```python
from build123d import *

# Parameters (mm, degrees)
BOSS_EXTRUDE1_DEPTH       = 35.56
CORTAR_EXTRUIR1_DEPTH     = 12.7
CORTAR_EXTRUIR2_DEPTH     = 12.7
CROQUIS4_R                = 6.35
CORTAR_EXTRUIR3_DEPTH     = 35.56
SIMETR_A7_COPY_1_SKETCH_R = 6.35
SIMETR_A7_COPY_1_DEPTH    = 35.56
REDONDEO1_R               = 17.78


with BuildPart() as part:
    # Sketch1 → Boss-Extrude1 (new body)
    with BuildSketch(Plane(origin=(0, 0, 0), x_dir=(1, 0, 0), z_dir=(0, 1, 0))):
        Polygon((47.97173767, 52.13499004), (20.15284418, 0), (47.971737664, -52.13499003), (16.598657301, -68.875462799), (0, -37.768156774), (-16.598657301, -68.875462799), (-32.285197483, -60.505226415), (-47.971737664, -52.13499003), (-20.15284418, 0), (-47.971737664, 52.13499003), (-32.285197483, 60.505226415), (-16.598657301, 68.875462799), (0, 37.768156774), (16.598657296, 68.875462789), (32.28519748, 60.505226416), align=None)
    extrude(amount=BOSS_EXTRUDE1_DEPTH)

    # Croquis2 → Cortar-Extruir1 (cut, symmetric)
    with BuildSketch(Plane(origin=(0, 0, 0), x_dir=(-0.470766951, 0, 0.882257603), z_dir=(-0.882257603, 0, -0.470766951))):
        with BuildLine():
            Line((55.88, 30.48), (68.58, 30.48))
            Line((68.58, 30.48), (68.58, 0))
            Line((68.58, 0), (43.18, 0))
            Line((43.18, 0), (43.18, 17.78))
            ThreePointArc((43.18, 17.78), (46.899743879, 26.760256121), (55.88, 30.48))
        make_face()
    cortar_extruir1 = extrude(amount=CORTAR_EXTRUIR1_DEPTH, both=True, mode=Mode.SUBTRACT)

    # Croquis3 → Cortar-Extruir2 (cut, symmetric)
    with BuildSketch(Plane(origin=(0, 0, 0), x_dir=(-0.470766951, 0, -0.882257603), z_dir=(0.882257603, 0, -0.470766951))):
        with BuildLine():
            Line((-55.88, 30.48), (-68.58, 30.48))
            Line((-68.58, 30.48), (-68.58, 0))
            Line((-68.58, 0), (-43.18, 0))
            Line((-43.18, 0), (-43.18, 17.78))
            ThreePointArc((-43.18, 17.78), (-46.899743879, 26.760256121), (-55.88, 30.48))
        make_face()
    cortar_extruir2 = extrude(amount=CORTAR_EXTRUIR2_DEPTH, both=True, mode=Mode.SUBTRACT)

    # Simetría1: Cortar-Extruir1, Cortar-Extruir2 across plane
    add(cortar_extruir1.mirror(Plane.XY), mode=Mode.SUBTRACT)
    add(cortar_extruir2.mirror(Plane.XY), mode=Mode.SUBTRACT)

    # Croquis4 → Cortar-Extruir3 (cut)
    with BuildSketch(Plane(origin=(-15.686540182, 0, -8.370236384), x_dir=(-0.470766951, 0, 0.882257603), z_dir=(-0.882257603, 0, -0.470766951))):
        with Locations((55.88, 17.78)):
            Circle(CROQUIS4_R)
    cortar_extruir3 = extrude(amount=-CORTAR_EXTRUIR3_DEPTH, mode=Mode.SUBTRACT)

    # Simetría2: Cortar-Extruir3 across plane
    add(cortar_extruir3.mirror(Plane(origin=(0, 0, 0), x_dir=(0, 0, 1), z_dir=(1, 0, 0))), mode=Mode.SUBTRACT)

    # Simetría7: Cortar-Extruir3 across plane
    add(cortar_extruir3.mirror(Plane.XY), mode=Mode.SUBTRACT)

    # Simetría7 copy 1 sketch → Simetría7 copy 1 (cut)
    with BuildSketch(Plane(origin=(15.686540182, 0, 8.370236384), x_dir=(0.470766951, 0, -0.882257603), z_dir=(0.882257603, 0, 0.470766951))):
        with Locations((55.88, 17.78)):
            Circle(SIMETR_A7_COPY_1_SKETCH_R)
    extrude(amount=-SIMETR_A7_COPY_1_DEPTH, mode=Mode.SUBTRACT)

    # Redondeo1
    redondeo1_edges = [part.edges().sort_by_distance(p)[0] for p in [
        (18.839591613, 0, 67.679714744),
        (-45.730803353, 0, 53.330738085),
        (-18.839591613, 0, -67.679714744),
        (45.730803357, 0, -53.330738094),
        (-18.839591613, 0, 67.679714744),
        (45.730803353, 0, 53.330738085),
        (-45.730803353, 0, -53.330738085),
        (18.839591608, 0, -67.679714736),
    ]]
    fillet(redondeo1_edges, radius=REDONDEO1_R)


solid = part.part
```
Read the model definition and answer for the solid it produces. Units are mm, in the model's axes. A direction names the side the tool comes from. Give positions to 0.01 mm unless a question says otherwise; leave off trailing zeros. Loops run counter-clockwise (first coordinate to the right, second up) from the corner with the lowest first, then second, coordinate; pieces in that order, holes last.
Item 1: The part is cut by section C-C (y = 3). Write down the section's boundary in (x, z).
Item 2: The part is cut by section B-B (z = 21). Write down the section's boundary in (x, y), and give its area (3 significant figures).
Item 3: For faces 1 (the cylindrical face through (43.38, 5.35, -48.84)), 2 (the cylindrical face through (42.635, 19.687, -47.453)), 3 (the flat face through (34.257, 17.531, -26.432)), 4 (the flat face through (6.57, 17.53, 50.08)), 5 (the cylindrical face through (-22.189, 26.661, -41.207)), determine the directions among +Z, -Z, +X, -X, +Y, -Y from which every point of the face is accessible in a straight line to the end or side of a thin tool.
Item 4: The mould has two halves that part along X. Classify faces 6 (the cylindrical face through (16.29, 5.07, 62.98)), 7 (the flat face through (29, 30.48, 55)), 8 (the cylindrical face through (-16.29, 5.07, -62.98)): released by +X, released by -X, zero draft, split by the parting line, or undercut.
Item 5: Find the intervals of material crossed by line 1 along X through (y, z) = (8.5, -46.5); line 2 along Z through (x, y) = (-18.5, 28); line 3 along X through (y, z) = (25.5, 44.5), in increasing order.
Item 6: The part is cut by section D-D (z = 58.5). Give the number of separate pieces and of enclosed holes in the cut face, and give its area (3 significant figures).
Item 7: Each of these flat-tipped pins is pushed along its axis until it touches: pin 1 Ø4 at (x, y) = (23.5, 5.5) entering from -Z; pin 2 Ø1 at (y, z) = (22, -5.5) entering from +X; pin 3 Ø18.5 at (x, z) = (-35.5, -49.5) entering from -Y; pin 4 Ø1 at (x, z) = (-29.5, 13.5) entering from -Y. Where does it stop, or does it pass through?
Item 8: The part is cut by section A-A (y = 32.5). Write down the section's boundary in (x, z) (3 decimals).
Taken from the geometry:
1. outline: (-44.25, -45.17) - (-39.77, -47.56) - (-31.53, -32.12) - (-9.12, -44.07) - (-17.36, -59.52) - (-12.88, -61.91) - (0, -37.77) - (12.88, -61.91) - (17.36, -59.52) - (9.12, -44.07) - (31.53, -32.12) - (39.77, -47.56) - (44.25, -45.17) - (20.15, 0) - (44.25, 45.17) - (39.77, 47.56) - (31.53, 32.12) - (9.12, 44.07) - (17.36, 59.52) - (12.88, 61.91) - (0, 37.77) - (-12.88, 61.91) - (-17.36, 59.52) - (-9.12, 44.07) - (-31.53, 32.12) - (-39.77, 47.56) - (-44.25, 45.17) - (-20.15, 0) - close
2. outline: (-31.36, 0) - (31.36, 0) - (31.36, 35.56) - (-31.36, 35.56) - close
2. area: 2,230 mm2
3. face 1: -Z, +X, -Y
3. face 2: none
3. face 3: +X, +Y, -Y
3. face 4: +Z, +Y, -Y
3. face 5: -Y
4. face 6: released by +X
4. face 7: undercut
4. face 8: released by -X
5. line 1: x = -44.96 to -39.21, -10.42 to -4.66, 4.66 to 10.42, 39.21 to 44.96
5. line 2: z = -67.86 to -61.65, -44.92 to 44.92, 61.65 to 67.86
5. line 3: x = -43.9 to -38.14, -13.88 to -3.59, 3.59 to 13.88, 38.14 to 43.9
6. separate pieces: 4
6. enclosed holes: 0
6. area: 451 mm2
7. pin 1: stops at z = -37.47
7. pin 2: stops at x = 23.35
7. pin 3: stops at y = 0.07
7. pin 4: passes through
8. outline: (-47.972, -52.135) - (-16.599, -68.875) - (0, -37.768) - (16.599, -68.875) - (47.972, -52.135) - (20.153, 0) - (47.972, 52.135) - (16.599, 68.875) - (0, 37.768) - (-16.599, 68.875) - (-47.972, 52.135) - (-20.153, 0) - close
